Autodesk Inventor part; units mm, degrees
ref_plane "XZ Plane" through (0, 0, 0) normal (0, 1, 0) x (-1, 0, 0)
ref_plane "XY Plane" through (0, 0, 0) normal (0, 0, 1) x (1, 0, 0)
sketch "Sketch1" plane through (0, 0, 0) normal (0, 1, 0) x (-1, 0, 0)
  line L0 (-177.8, 127) -> (-177.8, -127)
  line L1 (-177.8, -127) -> (177.8, -127)
  line L2 (177.8, -127) -> (177.8, 127)
  line L3 (177.8, 127) -> (-177.8, 127)
  line L4 (-177.8, 127) -> (177.8, -127) construction
  line L5 (-177.8, -127) -> (177.8, 127) construction
  point P0 (0, 0)
  dimension "d0" = 355.6
  dimension "d1" = 254
extrude "Extrusion1" add sketch "Sketch1" against normal blind 17.78
sketch "Sketch3" plane through (0, 0, 0) normal (0, 1, 0) x (1, 0, 0)
  line L0 (-177.8, -127) -> (-177.8, 127) construction
  line L1 (-177.8, 0) -> (177.8, 0) construction
  line L2 (177.8, 127) -> (177.8, -127) construction
  line L3 (-127, -25.4) -> (-123.825, -25.4)
  line L4 (-123.825, -25.4) -> (-123.825, 25.4)
  line L5 (-123.825, 25.4) -> (-127, 25.4)
  line L6 (-127, 25.4) -> (-127, -25.4)
  line L7 (-127, -25.4) -> (-123.825, 25.4) construction
  line L8 (-123.825, -25.4) -> (-127, 25.4) construction
  line L9 (-98.425, -25.4) -> (-95.25, -25.4)
  line L10 (-95.25, -25.4) -> (-95.25, 25.4)
  line L11 (-95.25, 25.4) -> (-98.425, 25.4)
  line L12 (-98.425, 25.4) -> (-98.425, -25.4)
  line L13 (-98.425, -25.4) -> (-95.25, 25.4) construction
  line L14 (-95.25, -25.4) -> (-98.425, 25.4) construction
  line L15 (-177.8, 127) -> (177.8, 127) construction
  line L16 (0, 127) -> (0, -127) construction
  line L17 (177.8, -127) -> (-177.8, -127) construction
  point P0 (0, 0)
  point P1 (-125.4125, 0)
  point P2 (-96.8375, 0)
  dimension "d4" = 50.8
  dimension "d5" = 3.175
  dimension "d6" = 50.8
  dimension "d7" = 25.4
extrude "Extrusion2" add sketch "Sketch3" along normal blind 50.8
sketch "Sketch4" plane through (-127, 0, -25.4) normal (-1, 0, 0) x (0, 0, 1)
  line L0 (25.4, 0) -> (25.4, 50.8) construction
  line L1 (50.8, 50.8) -> (0, 50.8) construction
  circle A0 centre (25.4, 25.4) radius 3.175
  dimension "d10" = 6.35
  dimension "d11" = 25.4
extrude "Extrusion3" cut sketch "Sketch4" against normal through all
mirror "Mirror2" about plane through (0, 0, 0) normal (1, 0, 0) of "Extrusion2", "Extrusion3"
equation "\"d0\" = plateWidth"
equation "\"d1\" = plateLength"
equation "\"d2\" = plateThickness"
equation "\"d4\" = bracketDistanceFromEdge"
equation "\"d5\" = bracketWidth"
equation "\"d6\" = bracketLength"
equation "\"d8\" = bracketHeight"
equation "\"d10\" = axelDiam"
equation "\"d11\" = axelHoleDistanceFromTopOfBracket"
equation "\"d12\" = bracketHeight"
equation "\"plateWidth\" = 355.6"
equation "\"plateLength\" = 254"
equation "\"plateThickness\" = 17.78"
equation "\"bracketDistanceFromEdge\" = 50.8"
equation "\"bracketWidth\" = 3.175"
equation "\"bracketHeight\" = 50.8"
equation "\"bracketLength\" = 50.8"
equation "\"axelDiam\" = 6.35"
equation "\"axelHoleDistanceFromTopOfBracket\" = 25.4"
properties part number "ExampleOfUsingSnowBlowerMotor"
Build history of the part. All positions in model axes, mm. A direction names the side the tool comes from. Give positions to 0.01 mm unless a question says otherwise; leave off trailing zeros. Loops run counter-clockwise (first coordinate to the right, second up) from the corner with the lowest first, then second, coordinate; pieces in that order, holes last. Notation, with made-up numbers: (38, 12) -> (70, 12) arc R20 cw to (70, 41) -> close; hole circle Ø1 at (45, 26). An arc over 180 degrees is marked (long way). One line per question, with ' | ' between items.
Q1. Drop flat-ended pins along their axis: pin 1 (1 mm diameter, centred on x = -124.5, y = 28, fed in from -Z); pin 2 (10 mm diameter, centred on x = -125, z = 80.5, fed in from +Y); pin 3 (5 mm diameter, centred on y = 12, z = 10.5, fed in from +X); pin 4 (12 mm diameter, centred on x = -135.5, y = 0.5, fed in from +Z). Give the stop position or say it passes through.
Filled sheet:
pin 1: stops at z = -25.4 | pin 2: stops at y = 0 | pin 3: stops at x = 127 | pin 4: stops at z = 127
Q2. Drill centre lines: line 1 along X through (y, z) = (3.5, 3.5) (3 decimals); line 2 along Y through (x, z) = (-125, 0) (3 decimals); line 3 along Z through (x, y) = (125.75, 25.4) (3 decimals). Where is each one in solid material? Low to high. Write a range as [from, to].
Filled sheet:
line 1: x = [-127, -123.825], [-98.425, -95.25], [95.25, 98.425], [123.825, 127] | line 2: y = [-17.78, 22.225], [28.575, 50.8] | line 3: z = [-25.4, -3.175], [3.175, 25.4]
Q3. Cut at B-B, the plane x = -64.5. Write the cut outline in (y, z).
Filled sheet:
outline: (-17.78, -127) -> (0, -127) -> (0, 127) -> (-17.78, 127) -> close
Q4. Tool access for faces 1 (the flat face through (-127, 31, 0)), 2 (the flat face through (2, -9, -127)), 3 (the flat face through (2, -17.78, 2)), 4 (the flat face through (98.425, 31, 0)), 5 (the flat face through (127, 31, 0)): list every direction of +Z, -Z, +X, -X, +Y, -Y with a clear straight run to the whole face (end or side of a thin tool).
Filled sheet:
face 1: +Z, -Z, -X, +Y | face 2: -Z, +X, -X, +Y, -Y | face 3: +Z, -Z, +X, -X, -Y | face 4: +Z, -Z, +Y | face 5: +Z, -Z, +X, +Y
Q5. Cut at C-C, the plane z = 42. Write the cut outline in (x, y), plus the area to 3 significant figures.
Filled sheet:
outline: (-177.8, -17.78) -> (177.8, -17.78) -> (177.8, 0) -> (-177.8, 0) -> close | area: 6,320 mm²
Q6. Cut at A-A, the plane y = 4.5. Write the cut outline in (x, z) (3 decimals).
Filled sheet:
outline: (-127, -25.4) -> (-123.825, -25.4) -> (-123.825, 25.4) -> (-127, 25.4) -> close; (-98.425, -25.4) -> (-95.25, -25.4) -> (-95.25, 25.4) -> (-98.425, 25.4) -> close; (95.25, -25.4) -> (98.425, -25.4) -> (98.425, 25.4) -> (95.25, 25.4) -> close; (123.825, -25.4) -> (127, -25.4) -> (127, 25.4) -> (123.825, 25.4) -> close
